from build123d import *

# Parameters (mm, degrees)
SKETCH1_W           = 91
SKETCH1_H           = 26
BOSS_EXTRUDE1_DEPTH = 5
SKETCH2_R           = 2.25
CUT_EXTRUDE1_DEPTH  = 2.5
SKETCH4_R           = 1.6
CUT_EXTRUDE3_DEPTH  = 3.5
SKETCH5_W           = 97
SKETCH5_H           = 32
SKETCH5_W_2         = 91
SKETCH5_H_2         = 26
BOSS_EXTRUDE2_DEPTH = 23
CUT_EXTRUDE4_REACH  = 34
SKETCH6_W           = 54
SKETCH6_H           = 7
SKETCH9_W           = 76
SKETCH9_H           = 5
BOSS_EXTRUDE3_DEPTH = 22.5
SKETCH10_R          = 2.25
CUT_EXTRUDE5_DEPTH  = 2.5
SKETCH11_R          = 1.6
CUT_EXTRUDE6_DEPTH  = 3.5
BOSS_EXTRUDE4_DEPTH = 35
CUT_EXTRUDE7_REACH  = 84
SKETCH13_R          = 1.6
CUT_EXTRUDE8_REACH  = 59.5
SKETCH14_R          = 1.6
SKETCH16_R          = 2.25
CUT_EXTRUDE10_DEPTH = 2.5
SKETCH17_R          = 2.5
SKETCH17_R_2        = 1.6
BOSS_EXTRUDE5_DEPTH = 1.3
SKETCH18_R          = 2.25
CUT_EXTRUDE11_DEPTH = 1.5


with BuildPart() as part:
    # Sketch1 → Boss-Extrude1 (new body)
    with BuildSketch(Plane(origin=(0, 0, 0), x_dir=(1, 0, 0), z_dir=(0, 1, 0))):
        with Locations((45.5, 13)):
            Rectangle(SKETCH1_W, SKETCH1_H)
    extrude(amount=BOSS_EXTRUDE1_DEPTH)

    # Sketch2 → Cut-Extrude1 (cut)
    with BuildSketch(Plane(origin=(0, 5, 0), x_dir=(1, 0, 0), z_dir=(0, 1, 0))):
        with Locations((2.5, 2.5)):
            Circle(SKETCH2_R)
        with Locations((88.5, 2.5)):
            Circle(SKETCH2_R)
        with Locations((29, 23.5)):
            Circle(SKETCH2_R)
    extrude(amount=-CUT_EXTRUDE1_DEPTH, mode=Mode.SUBTRACT)

    # Sketch4 → Cut-Extrude3 (cut, through all)
    with BuildSketch(Plane(origin=(0, 2.5, 0), x_dir=(1, 0, 0), z_dir=(0, 1, 0))):
        with Locations((2.5, 2.5)):
            Circle(SKETCH4_R)
        with Locations((29, 23.5)):
            Circle(SKETCH4_R)
        with Locations((88.5, 2.5)):
            Circle(SKETCH4_R)
    extrude(amount=-CUT_EXTRUDE3_DEPTH, mode=Mode.SUBTRACT)

    # Sketch5 → Boss-Extrude2 (add)
    with BuildSketch(Plane.XZ):
        with Locations((45.5, -13)):
            Rectangle(SKETCH5_W, SKETCH5_H)
        with Locations((45.5, -13)):
            Rectangle(SKETCH5_W_2, SKETCH5_H_2, mode=Mode.SUBTRACT)
    extrude(amount=-BOSS_EXTRUDE2_DEPTH)

    # Sketch6 → Cut-Extrude4 (cut, up to next)
    with BuildSketch(Plane.XY.offset(3), mode=Mode.PRIVATE) as cut_extrude4_sk1:
        with Locations((56, 11.5)):
            Rectangle(SKETCH6_W, SKETCH6_H)
    cut_extrude4_tool1 = extrude(cut_extrude4_sk1.sketch, amount=-CUT_EXTRUDE4_REACH, mode=Mode.PRIVATE) & part.part
    add(cut_extrude4_tool1.solids().sort_by_distance((56, 11.5, 3))[0], mode=Mode.SUBTRACT)

    # Sketch9 → Boss-Extrude3 (add)
    with BuildSketch(Plane(origin=(0, 0, -29), x_dir=(-1, 0, 0), z_dir=(0, 0, -1))):
        with Locations((-38, 2.5)):
            Rectangle(SKETCH9_W, SKETCH9_H)
    extrude(amount=BOSS_EXTRUDE3_DEPTH)

    # Sketch10 → Cut-Extrude5 (cut)
    with BuildSketch(Plane(origin=(0, 5, 0), x_dir=(1, 0, 0), z_dir=(0, 1, 0))):
        with Locations((29, 49)):
            Circle(SKETCH10_R)
    extrude(amount=-CUT_EXTRUDE5_DEPTH, mode=Mode.SUBTRACT)

    # Sketch11 → Cut-Extrude6 (cut, through all)
    with BuildSketch(Plane(origin=(0, 2.5, 0), x_dir=(1, 0, 0), z_dir=(0, 1, 0))):
        with Locations((29, 49)):
            Circle(SKETCH11_R)
    extrude(amount=-CUT_EXTRUDE6_DEPTH, mode=Mode.SUBTRACT)

    # Sketch12 → Boss-Extrude4 (add)
    with BuildSketch(Plane.XZ):
        Polygon((0, -29), (-3, -29), (-3, -54.5), (0, -54.5), (79, -54.5), (79, -51.5), (79, -29), (76, -29), (76, -51.5), (0, -51.5), align=None)
    extrude(amount=-BOSS_EXTRUDE4_DEPTH)

    # Sketch13 → Cut-Extrude7 (cut, up to next)
    with BuildSketch(Plane(origin=(79, 0, 0), x_dir=(0, 0, -1), z_dir=(1, 0, 0)), mode=Mode.PRIVATE) as cut_extrude7_sk1:
        with Locations((31.5, 10)):
            Circle(SKETCH13_R)
    cut_extrude7_tool1 = extrude(cut_extrude7_sk1.sketch, amount=-CUT_EXTRUDE7_REACH, mode=Mode.PRIVATE) & part.part
    add(cut_extrude7_tool1.solids().sort_by_distance((79, 10, -31.5))[0], mode=Mode.SUBTRACT)

    # Sketch14 → Cut-Extrude8 (cut, up to next)
    with BuildSketch(Plane(origin=(0, 0, -54.5), x_dir=(-1, 0, 0), z_dir=(0, 0, -1)), mode=Mode.PRIVATE) as cut_extrude8_sk1:
        with Locations((-54.45, 7.5)):
            Circle(SKETCH14_R)
    cut_extrude8_tool1 = extrude(cut_extrude8_sk1.sketch, amount=-CUT_EXTRUDE8_REACH, mode=Mode.PRIVATE) & part.part
    add(cut_extrude8_tool1.solids().sort_by_distance((54.45, 7.5, -54.5))[0], mode=Mode.SUBTRACT)
    # Sketch14 → Cut-Extrude8 (cut, up to next)
    with BuildSketch(Plane(origin=(0, 0, -54.5), x_dir=(-1, 0, 0), z_dir=(0, 0, -1)), mode=Mode.PRIVATE) as cut_extrude8_sk2:
        with Locations((-2.55, 12.2)):
            Circle(SKETCH14_R)
    cut_extrude8_tool2 = extrude(cut_extrude8_sk2.sketch, amount=-CUT_EXTRUDE8_REACH, mode=Mode.PRIVATE) & part.part
    add(cut_extrude8_tool2.solids().sort_by_distance((2.55, 12.2, -54.5))[0], mode=Mode.SUBTRACT)

    # Sketch16 → Cut-Extrude10 (cut)
    with BuildSketch(Plane.XY.offset(-51.5)):
        with Locations((2.55, 12.2)):
            Circle(SKETCH16_R)
        with Locations((54.45, 7.5)):
            Circle(SKETCH16_R)
    extrude(amount=-CUT_EXTRUDE10_DEPTH, mode=Mode.SUBTRACT)

    # Sketch17 → Boss-Extrude5 (add)
    with BuildSketch(Plane(origin=(0, 0, -54.5), x_dir=(-1, 0, 0), z_dir=(0, 0, -1))):
        with Locations((-54.45, 7.5)):
            Circle(SKETCH17_R)
        with Locations((-54.45, 7.5)):
            Circle(SKETCH17_R_2, mode=Mode.SUBTRACT)
        with Locations((-2.55, 12.2)):
            Circle(SKETCH17_R)
        with Locations((-2.55, 12.2)):
            Circle(SKETCH17_R_2, mode=Mode.SUBTRACT)
    extrude(amount=BOSS_EXTRUDE5_DEPTH)

    # Sketch18 → Cut-Extrude11 (cut)
    with BuildSketch(Plane.ZY.offset(-76)):
        with Locations((-31.5, 10)):
            Circle(SKETCH18_R)
    extrude(amount=-CUT_EXTRUDE11_DEPTH, mode=Mode.SUBTRACT)


solid = part.part
Build history of the part. All positions in model axes, mm. A direction names the side the tool comes from. Coordinates: 2 decimals unless noted, no trailing zeros. Order: outer loops, then holes, each group sorted by start corner. A loop starts at its lowest first (then second) coordinate and runs counter-clockwise, first axis right, second up. Notation, with made-up numbers: M 77,89 L 102,89 A24 cw 102,120 Z; hole C 0,27.5 d6. An arc over 180 degrees is marked long. One line per question, with ' | ' between items. Start each with the question number.
Q1. Saw through at B-B (x = 54.45). List the corners of the cut face in (y, z).
Q2. Saw through at C-C (y = 20.5). List the corners of the cut face in (x, z).
Q3. Probe L1, parallel to Z at x = 68.5, y = 22; L2, parallel to X at y = 1.1, z = -49; L3, parallel to Z at x = 29, y = 3. List the from-to ranges inside material, lowest first. Write a range as from..to.
Q4. Saw through at D-D (z = -31.5). List the corners of the cut face in (x, y), then the cut area to 3 significant figures.
Q5. Saw through at A-A (z = -23.5). List the corners of the cut face in (x, y).
Q6. Flat gauge pins, fed straight in: pin 1 Ø6 at (x, z) = (29, -23.5) entering from +Y; pin 2 Ø1.5 at (x, z) = (9.5, -36) entering from +Y; pin 3 Ø17.5 at (x, y) = (40, 15.5) entering from -Z. Where does each tip first touch, or does it go through?
Q7. Two-plate mould, pull along X, no slides. Class faces 1 (the face through (86, 11, -29)), 2 (the face through (39, 20, -51.5)), 3 (the face through (94, 11, -13)): +X half, -X half, draft (parallel to the pull), parting line (faces both ways), or undercut.
Q8. 3-axis set-ups, long thin cutter, end or side, ignore diameter. For faces 4 (the face through (83, 11, 2)), 5 (the face through (89.5, 2.5, -1)), 6 (the face through (86.9, 1.27, -2.57)), 7 (the face through (3, 14, -54)), 8 (the face through (78, 29, -29)): which of +Z, -Z, +X, -X, +Y, -Y reach the whole face in a straight line?
Check values:
1) outline: M 0,-54.5 L 5,-54.5 L 5,-55.8 L 5.9,-55.8 L 5.9,-54 L 5.25,-54 L 5.25,-51.5 L 5,-51.5 L 5,-29 L 23,-29 L 23,-26 L 5,-26 L 5,0 L 8,0 L 8,3 L 0,3 Z; M 9.1,-55.8 L 10,-55.8 L 10,-54.5 L 35,-54.5 L 35,-51.5 L 9.75,-51.5 L 9.75,-54 L 9.1,-54 Z; M 15,0 L 23,0 L 23,3 L 15,3 Z
2) outline: M -3,-54.5 L 79,-54.5 L 79,-29 L 94,-29 L 94,3 L -3,3 Z; hole M 0,-51.5 L 76,-51.5 L 76,-29 L 0,-29 Z; hole M 0,-26 L 91,-26 L 91,0 L 0,0 Z
3) L1: z = -54.5..-51.5, -29..-26, 0..3 | L2: x = -3..27.4, 30.6..79 | L3: z = -54.5..-51.25, -46.75..-25.75, -21.25..3
4) outline: M -3,0 L 79,0 L 79,8.4 L 77.5,8.4 L 77.5,7.75 L 76,7.75 L 76,5 L 0,5 L 0,35 L -3,35 Z; M 76,12.25 L 77.5,12.25 L 77.5,11.6 L 79,11.6 L 79,35 L 76,35 Z | area: 578 mm2
5) outline: M -3,0 L 27.4,0 L 27.4,2.5 L 26.75,2.5 L 26.75,5 L 0,5 L 0,23 L -3,23 Z; M 30.6,0 L 94,0 L 94,23 L 91,23 L 91,5 L 31.25,5 L 31.25,2.5 L 30.6,2.5 Z
6) pin 1: stops at y = 23 | pin 2: stops at y = 5 | pin 3: stops at z = -54.5
7) face 1: draft | face 2: undercut | face 3: +X half
8) face 4: +Z | face 5: +Y | face 6: +Y, -Y | face 7: none | face 8: +Z, +X, -X, +Y
